Design review of the part built by this model. Coordinates are the model's own, in mm. Give positions to 0.01 mm unless a question says otherwise; leave off trailing zeros. Order: outer loops, then holes, each group sorted by start corner. A loop starts at its lowest first (then second) coordinate and runs counter-clockwise, first axis right, second up.
```python
from build123d import *

# Parameters (mm, degrees)
SKETCH1_R                 = 10
SKETCH1_R_2               = 8
BOSS_EXTRUDE1_DEPTH       = 5
SKETCH2_W                 = 10
SKETCH2_H                 = 5
BOSS_EXTRUDE2_DEPTH       = 250
BOSS_EXTRUDE3_START       = -5
BOSS_EXTRUDE3_DEPTH       = 5
BOSS_EXTRUDE4_START       = 20
SKETCH5_R                 = 8
BOSS_EXTRUDE4_DEPTH       = 20
CUT_EXTRUDE1_DEPTH        = 257.953303151
CUT_EXTRUDE1_DEPTH_BACK   = 257.953303151
BOSS_EXTRUDE5_START       = -2.5
SKETCH7_W                 = 5
SKETCH7_H                 = 255
BOSS_EXTRUDE5_DEPTH       = 5
SKETCH9_W                 = 50
SKETCH9_H                 = 10
BOSS_EXTRUDE6_DEPTH       = 2.5
BOSS_EXTRUDE7_START       = -5
SKETCH9_2_W               = 50
SKETCH9_2_H               = 10
BOSS_EXTRUDE7_DEPTH       = 2.5
SKETCH10_R                = 4
BOSS_EXTRUDE8_DEPTH       = 15
LPATTERN1_COUNT           = 2
LPATTERN1_PITCH           = 160
LPATTERN2_COUNT           = 2
LPATTERN2_PITCH           = 20
LPATTERN3_COPY_1_SKETCH_W = 50
LPATTERN3_COPY_1_SKETCH_H = 10
LPATTERN3_COPY_1_DEPTH    = 2.5
LPATTERN3_START           = -5
LPATTERN3_COPY_2_SKETCH_W = 50
LPATTERN3_COPY_2_SKETCH_H = 10
LPATTERN3_COPY_2_DEPTH    = 2.5
LPATTERN3_COPY_3_SKETCH_R = 4
LPATTERN3_COPY_3_DEPTH    = 15
LPATTERN3_COPY_4_SKETCH_W = 50
LPATTERN3_COPY_4_SKETCH_H = 10
LPATTERN3_COPY_4_DEPTH    = 2.5
LPATTERN3_COPY_5_SKETCH_W = 50
LPATTERN3_COPY_5_SKETCH_H = 10
LPATTERN3_COPY_5_DEPTH    = 2.5
LPATTERN3_COPY_6_SKETCH_R = 4
LPATTERN3_COPY_6_DEPTH    = 15
BOSS_EXTRUDE9_START       = 25
SKETCH11_R                = 4
BOSS_EXTRUDE9_DEPTH       = 25
SKETCH12_W                = 10
SKETCH12_H                = 30
BOSS_EXTRUDE10_DEPTH      = 2.5
BOSS_EXTRUDE11_START      = 35
SKETCH11_2_R              = 4
BOSS_EXTRUDE11_DEPTH      = 7.5


with BuildPart() as part:
    # Sketch1 → Boss-Extrude1 (new body)
    # profile 1 of 3: a face of its own
    with BuildSketch(Plane.XY):
        Circle(SKETCH1_R)
        Circle(SKETCH1_R_2, mode=Mode.SUBTRACT)
    # profile 2 of 3: a face of its own
    with BuildSketch(Plane.XY):
        with BuildLine():
            ThreePointArc((-5, 8.660254038), (-2.588190451, 9.659258263), (0, 10))
            Line((0, 10), (0, 30))
            Line((0, 30), (-5, 30))
            Line((-5, 30), (-5, 8.660254038))
        make_face()
    # profile 3 of 3: a face of its own
    with BuildSketch(Plane.XY):
        with BuildLine():
            Line((0, 30), (0, 10))
            ThreePointArc((0, 10), (2.588190451, 9.659258263), (5, 8.660254038))
            Line((5, 8.660254038), (5, 30))
            Line((5, 30), (0, 30))
        make_face()
    extrude(amount=BOSS_EXTRUDE1_DEPTH)

    # Sketch2 → Boss-Extrude2 (add)
    with BuildSketch(Plane.XY.offset(5)):
        with Locations((0, 27.5)):
            Rectangle(SKETCH2_W, SKETCH2_H)
    extrude(amount=BOSS_EXTRUDE2_DEPTH)

    # Sketch4 → Boss-Extrude3 (add)
    with BuildSketch(Plane.XY.offset(255).offset(BOSS_EXTRUDE3_START)):
        with BuildLine():
            Line((-5, 25), (5, 25))
            Line((5, 25), (5, 6.244997998))
            ThreePointArc((5, 6.244997998), (0, -8), (-5, 6.244997998))
            Line((-5, 6.244997998), (-5, 25))
        make_face()
    extrude(amount=BOSS_EXTRUDE3_DEPTH)

    # Sketch5 → Boss-Extrude4 (add)
    with BuildSketch(Plane(origin=(0, 0, 250), x_dir=(-1, 0, 0), z_dir=(0, 0, -1)).offset(BOSS_EXTRUDE4_START)):
        with Locations(Location((0, 0, 0), (0, 0, 180))):
            Circle(SKETCH5_R)
    extrude(amount=-BOSS_EXTRUDE4_DEPTH)

    # Sketch6 → Cut-Extrude1 (cut, two sides: drawn at the far end of the back side and taken through both)
    with BuildSketch(Plane(origin=(0, 0, 0), x_dir=(0, 0, -1), z_dir=(1, 0, 0)).offset(-CUT_EXTRUDE1_DEPTH_BACK)):
        Polygon((-243.585291862, 8.659957716), (-248.585291862, 8.659957716), (-239.925334146, 0), (-238.509860061, -1.415474085), (-233.925334146, -1.415474085), (-233.925334146, 1.415474085), (-236.340808231, 1.415474085), align=None)
    extrude(amount=CUT_EXTRUDE1_DEPTH + CUT_EXTRUDE1_DEPTH_BACK, mode=Mode.SUBTRACT)

    # Sketch7 → Boss-Extrude5 (add, symmetric)
    with BuildSketch(Plane.XZ.offset(-25).offset(BOSS_EXTRUDE5_START)):
        with Locations((0, 127.5)):
            Rectangle(SKETCH7_W, SKETCH7_H)
    extrude(amount=BOSS_EXTRUDE5_DEPTH, both=True)

    # Sketch9 → Boss-Extrude6 (add)
    with BuildSketch(Plane(origin=(0, 30, 0), x_dir=(1, 0, 0), z_dir=(0, 1, 0))):
        with Locations((0, -73.565096755)):
            Rectangle(SKETCH9_W, SKETCH9_H)
    boss_extrude6 = extrude(amount=BOSS_EXTRUDE6_DEPTH)

    # Sketch9<2> → Boss-Extrude7 (add)
    with BuildSketch(Plane(origin=(0, 30, 0), x_dir=(1, 0, 0), z_dir=(0, 1, 0)).offset(BOSS_EXTRUDE7_START)):
        with Locations((0, -73.565096755)):
            Rectangle(SKETCH9_2_W, SKETCH9_2_H)
    boss_extrude7 = extrude(amount=-BOSS_EXTRUDE7_DEPTH)

    # Sketch10 → Boss-Extrude8 (add)
    with BuildSketch(Plane(origin=(0, 25, 0), x_dir=(1, 0, 0), z_dir=(0, 1, 0))):
        with Locations(Location((20, -73.565096755, 0), (0, 0, 180))):
            Circle(SKETCH10_R)
        with Locations(Location((-20, -73.565096755, 0), (0, 0, 180))):
            Circle(SKETCH10_R)
    boss_extrude8 = extrude(amount=BOSS_EXTRUDE8_DEPTH)

    # LPattern1: Boss-Extrude6, Boss-Extrude7, Boss-Extrude8 ×2
    with Locations(*[(0, 0, i * LPATTERN1_PITCH) for i in range(1, LPATTERN1_COUNT)]):
        add(boss_extrude6)
        add(boss_extrude7)
        add(boss_extrude8)

    # LPattern2: Boss-Extrude6, Boss-Extrude7, Boss-Extrude8 ×2
    with Locations(*[(0, 0, -i * LPATTERN2_PITCH) for i in range(1, LPATTERN2_COUNT)]):
        add(boss_extrude6)
        add(boss_extrude7)
        add(boss_extrude8)

    # LPattern3 copy 1 sketch → LPattern3 copy 1 (add)
    with BuildSketch(Plane(origin=(0, 30, 140), x_dir=(1, 0, 0), z_dir=(0, 1, 0))):
        with Locations((0, -73.565096755)):
            Rectangle(LPATTERN3_COPY_1_SKETCH_W, LPATTERN3_COPY_1_SKETCH_H)
    extrude(amount=LPATTERN3_COPY_1_DEPTH)

    # LPattern3 copy 2 sketch → LPattern3 copy 2 (add)
    with BuildSketch(Plane(origin=(0, 30, 140), x_dir=(1, 0, 0), z_dir=(0, 1, 0)).offset(LPATTERN3_START)):
        with Locations((0, -73.565096755)):
            Rectangle(LPATTERN3_COPY_2_SKETCH_W, LPATTERN3_COPY_2_SKETCH_H)
    extrude(amount=-LPATTERN3_COPY_2_DEPTH)

    # LPattern3 copy 3 sketch → LPattern3 copy 3 (add)
    with BuildSketch(Plane(origin=(0, 25, 140), x_dir=(1, 0, 0), z_dir=(0, 1, 0))):
        with Locations(Location((20, -73.565096755, 0), (0, 0, 180))):
            Circle(LPATTERN3_COPY_3_SKETCH_R)
        with Locations(Location((-20, -73.565096755, 0), (0, 0, 180))):
            Circle(LPATTERN3_COPY_3_SKETCH_R)
    extrude(amount=LPATTERN3_COPY_3_DEPTH)

    # LPattern3 copy 4 sketch → LPattern3 copy 4 (add)
    with BuildSketch(Plane(origin=(0, 30, -20), x_dir=(1, 0, 0), z_dir=(0, 1, 0))):
        with Locations((0, -73.565096755)):
            Rectangle(LPATTERN3_COPY_4_SKETCH_W, LPATTERN3_COPY_4_SKETCH_H)
    extrude(amount=LPATTERN3_COPY_4_DEPTH)

    # LPattern3 copy 5 sketch → LPattern3 copy 5 (add)
    with BuildSketch(Plane(origin=(0, 30, -20), x_dir=(1, 0, 0), z_dir=(0, 1, 0)).offset(LPATTERN3_START)):
        with Locations((0, -73.565096755)):
            Rectangle(LPATTERN3_COPY_5_SKETCH_W, LPATTERN3_COPY_5_SKETCH_H)
    extrude(amount=-LPATTERN3_COPY_5_DEPTH)

    # LPattern3 copy 6 sketch → LPattern3 copy 6 (add)
    with BuildSketch(Plane(origin=(0, 25, -20), x_dir=(1, 0, 0), z_dir=(0, 1, 0))):
        with Locations(Location((20, -73.565096755, 0), (0, 0, 180))):
            Circle(LPATTERN3_COPY_6_SKETCH_R)
        with Locations(Location((-20, -73.565096755, 0), (0, 0, 180))):
            Circle(LPATTERN3_COPY_6_SKETCH_R)
    extrude(amount=LPATTERN3_COPY_6_DEPTH)

    # Sketch11 → Boss-Extrude9 (add)
    with BuildSketch(Plane.XZ.offset(-22.5).offset(BOSS_EXTRUDE9_START)):
        with Locations(Location((-20, 73.565096755, 0), (0, 0, 180))):
            Circle(SKETCH11_R)
        with Locations(Location((20, 73.565096755, 0), (0, 0, 180))):
            Circle(SKETCH11_R)
        with Locations(Location((20, 53.565096755, 0), (0, 0, 180))):
            Circle(SKETCH11_R)
        with Locations(Location((-20, 53.565096755, 0), (0, 0, 180))):
            Circle(SKETCH11_R)
    extrude(amount=-BOSS_EXTRUDE9_DEPTH)

    # Sketch12 → Boss-Extrude10 (add)
    with BuildSketch(Plane.XZ.offset(2.5)):
        with Locations((20, 63.565096755)):
            Rectangle(SKETCH12_W, SKETCH12_H)
        with Locations((-20, 63.565096755)):
            Rectangle(SKETCH12_W, SKETCH12_H)
    extrude(amount=BOSS_EXTRUDE10_DEPTH)

    # Sketch11<2> → Boss-Extrude11 (add)
    with BuildSketch(Plane.XZ.offset(-22.5).offset(BOSS_EXTRUDE11_START)):
        with Locations(Location((-20, 73.565096755, 0), (0, 0, 180))):
            Circle(SKETCH11_2_R)
        with Locations(Location((20, 73.565096755, 0), (0, 0, 180))):
            Circle(SKETCH11_2_R)
        with Locations(Location((20, 53.565096755, 0), (0, 0, 180))):
            Circle(SKETCH11_2_R)
        with Locations(Location((-20, 53.565096755, 0), (0, 0, 180))):
            Circle(SKETCH11_2_R)
    extrude(amount=-BOSS_EXTRUDE11_DEPTH)


solid = part.part
```
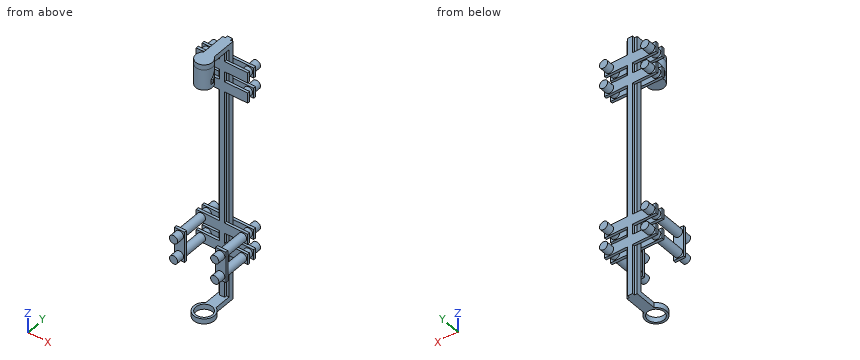
1. For line 1 along Z through (x, y) = (-12, 23); line 2 along Z through (x, y) = (20, 13); line 3 along Y through (x, z) = (0, 3.15), list the stretches that pass through material, from the lowest coordinate up.
Recorded:
line 1: z = 48.57 to 58.57, 68.57 to 78.57, 208.57 to 218.57, 228.57 to 238.57
line 2: z = 49.57 to 57.57, 69.57 to 77.57
line 3: y = -10 to -8, 8 to 32.5
2. For pin 1 (1.5 mm diameter, centred on x = -18.5, y = 25.5, fed in from +Z); pin 2 (2 mm diameter, centred on y = 23.5, z = 175.5, fed in from -X); pin 3 (11 mm diameter, centred on x = 10.5, z = 72.5, fed in from +Y), all flat-tipped, find the tip position at first contact; note any pin that passes through.
Recorded:
pin 1: stops at z = 238.57
pin 2: stops at x = -2.5
pin 3: stops at y = 32.5
3. Take a section at B-B (x = -20). State how many separate pieces and enclosed holes the cut face has, then the cut area to 4 significant figures.
Recorded:
separate pieces: 3
enclosed holes: 0
area: 1,195 mm2
4. Take a section at C-C (y = 15.5). State the section outline as (x, z) points.
Recorded:
outline: circle Ø8 at (-20, 53.57); circle Ø8 at (-20, 73.57); (-5, 0) - (5, 0) - (5, 5) - (-5, 5) - close; (-5, 250) - (5, 250) - (5, 255) - (-5, 255) - close; circle Ø8 at (20, 53.57); circle Ø8 at (20, 73.57)
5. Take a section at A-A (x = 0). State the section outline as (y, z) points.
Recorded:
outline: (-10, 0) - (-8, 0) - (-8, 5) - (-10, 5) - close; (-8, 230) - (8, 230) - (8, 242.93) - (1.42, 236.34) - (1.42, 233.93) - (-1.42, 233.93) - (-1.42, 238.51) - (8, 247.93) - (8, 250) - (22.5, 250) - (22.5, 5) - (8, 5) - (8, 0) - (32.5, 0) - (32.5, 255) - (-8, 255) - close
